The model under review builds one solid part; all positions refer to its coordinate system, in mm. Face numbers are marked on the shaded views. A direction names the side the tool comes from. Give positions to 0.01 mm unless a question says otherwise; leave off trailing zeros. Loops run counter-clockwise (first coordinate to the right, second up) from the corner with the lowest first, then second, coordinate; pieces in that order, holes last. Notation, with made-up numbers: (-31, 18.5) - (8, 18.5) arc R14 cw to (8, 42.5) - close; hole circle Ø7 at (81, 22.25). An arc over 180 degrees is marked (long way). Return JSON: item names as keys, results as strings. Group by question number.
from build123d import *

# Parameters (mm, degrees)
F0_R     = 12.7
F0_R_2   = 3
F1_DEPTH = 10
F2_R     = 12.7
F2_R_2   = 11.7
F3_DEPTH = 7


# Not quite as in the source:
# - a fillet or chamfer that OpenCascade refuses, or shapes differently, is made with other operations: its cross-section is extruded or revolved along the edge and cut away or added


with BuildPart() as f1:
    # F0 (on Top) → F1 (new body)
    with BuildSketch(Plane.XY):
        with Locations((0.256980346, -0.0691873614)):
            Circle(F0_R)
        with Locations((0.256980346, -8.3191873614)):
            Circle(F0_R_2, mode=Mode.SUBTRACT)
        with Locations((-7.993019654, -0.0691873614)):
            Circle(F0_R_2, mode=Mode.SUBTRACT)
        with Locations((0.256980346, -0.0691873614)):
            Circle(F0_R_2, mode=Mode.SUBTRACT)
        with Locations((8.506980346, -0.0691873614)):
            Circle(F0_R_2, mode=Mode.SUBTRACT)
        with Locations((0.256980346, 8.1808126386)):
            Circle(F0_R_2, mode=Mode.SUBTRACT)
    extrude(amount=F1_DEPTH)

    # F2 (on face) → F3 (cut)
    with BuildSketch(Plane(origin=(0, 0, 0), x_dir=(1, 0, 0), z_dir=(0, 0, -1))):
        with Locations((0.256980346, 0.0691873614)):
            Circle(F2_R)
        with Locations((0.256980346, 0.0691873614)):
            Circle(F2_R_2, mode=Mode.SUBTRACT)
    extrude(amount=-F3_DEPTH, mode=Mode.SUBTRACT)

    # F4: chamfer of 0.5 on 2 edges, made by hand

    # F4_s1 → F4_t2 (revolve, cut)
    with BuildSketch(Plane.XZ.offset(0.0691873614)):
        Polygon((12.956980346, 9.5), (12.456980346, 10), (12.956980346, 10), align=None)
    revolve(axis=Axis((0.256980346, -0.0691873614, 10), (0, 0, 1)), mode=Mode.SUBTRACT)

    # F4_s3 → F4_t4 (revolve, cut)
    with BuildSketch(Plane.XZ.offset(0.0691873614)):
        Polygon((11.956980346, 0.5), (11.456980346, 0), (11.956980346, 0), align=None)
    revolve(axis=Axis((0.256980346, -0.0691873614, 0), (0, 0, -1)), mode=Mode.SUBTRACT)


solid = f1.part
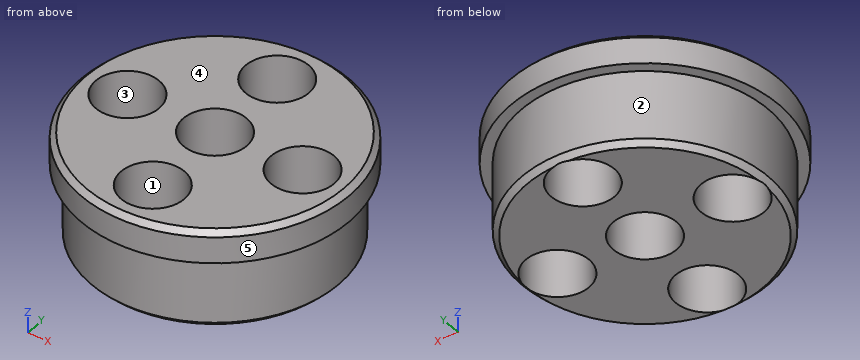
Item 1: Take a section at D-D (z = 3). State the section outline as (x, y) points, then the cut area to 3 significant figures.
Item 2: Tool access review of the marked faces 1 and 2: name each direction out of +Z, -Z, +X, -X, +Y, -Y from which nothing blocks a thin tool from reaching the whole face with its end or side.
Item 3: Take a section at B-B (x = -1). State how many separate pieces and enclosed holes the cut face has, then the cut area to 3 significant figures.
Item 4: Mouldability with a two-part tool opening along Y and no side actions: class the marked faces 3, 4 and 5 as +Y half, -Y half, draft (parallel to the pull), parting line (faces both ways), or undercut.
Item 5: Take a section at A-A (z = 8.5). State the section outline as (x, y) points, then the cut area to 3 significant figures.
Item 6: For P1, Ø1, axis at x = 10.5, y = -5, coming from the -Z side; P2, Ø3, axis at y = 1.5, z = 4.5, coming from the -X side; P3, Ø1, axis at x = -0.5, z = 6, coming from the +Y side; P4, Ø1.5, axis at x = -5, z = 8, coming from the -Y side, all flat-tipped, find the tip position at first contact; note any pin that passes through.
Item 7: For L1, parallel to X at y = -1.5, z = 3.75; L2, parallel to X at y = -2.75, z = 0.5; L3, parallel to Y at x = -1.75, z = 0.5, list the stretches that pass through material, from the lowest coordinate up. Write a range as from..to.
Check sheet entries:
{
 "1": {"outline": "circle Ø23.4 at (0.26, -0.07); hole circle Ø6 at (-7.99, -0.07); hole circle Ø6 at (0.26, -8.32); hole circle Ø6 at (0.26, -0.07); hole circle Ø6 at (0.26, 8.18); hole circle Ø6 at (8.51, -0.07)", "area": "289 mm^2"},
 "2": {"face 1": "+Z, -Z", "face 2": "-Z"},
 "3": {"separate pieces": "4", "enclosed holes": "0", "area": "74.7 mm^2"},
 "4": {"face 3": "undercut", "face 4": "draft", "face 5": "parting line"},
 "5": {"outline": "circle Ø25.4 at (0.26, -0.07); hole circle Ø6 at (-7.99, -0.07); hole circle Ø6 at (0.26, -8.32); hole circle Ø6 at (0.26, -0.07); hole circle Ø6 at (0.26, 8.18); hole circle Ø6 at (8.51, -0.07)", "area": "365 mm^2"},
 "6": {"P1": "stops at z = 0", "P2": "stops at x = -11.44", "P3": "stops at y = 11.63", "P4": "stops at y = -11.94"},
 "7": {"L1": "x = -11.36..-10.63, -5.36..-2.38, 2.89..5.87, 11.14..11.87", "L2": "x = -11.13..-9.34, -6.65..-1.09, 1.6..7.16, 9.85..11.65", "L3": "y = -11.6..-10.55, -6.09..-2.3, 2.16..5.95, 10.41..11.46"}
}
